The model under review builds one solid part; all positions refer to its coordinate system, in mm. A direction names the side the tool comes from. Give positions to 0.01 mm unless a question says otherwise; leave off trailing zeros. Write each loop counter-clockwise with the first axis right and the second up, starting at its lowest first coordinate (ties: lowest second). Pieces come first, ordered by that corner, then holes. Notation, with made-up numbers: (-25.75, 88) - (-18.75, 88) arc R20 ccw to (-18.75, 108) - close; hole circle Ø6 at (2.25, -25.75). An arc over 180 degrees is marked (long way). Write item = value, one per line.
```python
from build123d import *

# Parameters (mm, degrees)
F0_R     = 50.8
F0_R_2   = 47.752
F1_DEPTH = 34.036
F3_R     = 2.778125
F4_DEPTH = 12.7
F6_COUNT = 3
F6_ANGLE = 240


with BuildPart() as f1:
    # F0 (on Right) → F1 (new body, symmetric)
    with BuildSketch(Plane.YZ):
        Circle(F0_R)
        Circle(F0_R_2, mode=Mode.SUBTRACT)
    extrude(amount=F1_DEPTH, both=True)


with BuildPart() as f4:
    # F3 (on offset) → F4 (new body, symmetric)
    with BuildSketch(Plane.XY.offset(50.8)):
        with Locations((-28.575, 0)):
            Circle(F3_R)
        with Locations((28.575, 0)):
            Circle(F3_R)
    extrude(amount=F4_DEPTH, both=True)


with BuildPart() as f6_1:
    # F6: instance of F4
    add(f4.part.rotate(Axis((2.265271, 0, 0), (1, 0, 0)), 1 * F6_ANGLE / (F6_COUNT - 1)))


with BuildPart() as f6_2:
    # F6: instance of F4
    add(f4.part.rotate(Axis((2.265271, 0, 0), (1, 0, 0)), 2 * F6_ANGLE / (F6_COUNT - 1)))


with BuildPart() as f1_1:
    add(f1.part)

    # F7: cut F4, F6_2, F6_1
    add(f4.part, mode=Mode.SUBTRACT)
    add(f6_2.part, mode=Mode.SUBTRACT)
    add(f6_1.part, mode=Mode.SUBTRACT)


solid = f1_1.part
```
1. For line 1 (X direction, y = 0, z = 48.7); line 2 (Z direction, x = -12.5, y = 0); line 3 (Z direction, x = 17, y = -1.5), list the stretches that pass through material, from the lowest coordinate up. Write a range as from..to.
Findings below:
line_1 = -34.04..-31.35, -25.8..25.8, 31.35..34.04
line_2 = -50.8..-47.75, 47.75..50.8
line_3 = -50.78..-47.73, 47.73..50.78
2. Insertion check: P1, Ø1.5, axis at x = -13, y = 17.5, coming from the -Z side; P2, Ø5, axis at x = -10.5, y = -4, coming from the +Z side; P3, Ø10, axis at x = -2.5, z = -16, coming from the +Y side. Each pin has a flat end and moves straight along its axis. Give the tip position at first contact, or say it passes through.
Findings below:
P1 = -47.96
P2 = 50.78
P3 = 49.59
3. Take a section at B-B on y = 0. Give the boundary of the cut face in (x, z).
Findings below:
outline = (-34.04, -50.8) - (34.04, -50.8) - (34.04, -47.75) - (-34.04, -47.75) - close; (-34.04, 47.75) - (-31.35, 47.75) - (-31.35, 50.8) - (-34.04, 50.8) - close; (-25.8, 47.75) - (25.8, 47.75) - (25.8, 50.8) - (-25.8, 50.8) - close; (31.35, 47.75) - (34.04, 47.75) - (34.04, 50.8) - (31.35, 50.8) - close
4. Take a section at C-C on y = -35. Give the boundary of the cut face in (x, z).
Findings below:
outline = (-34.04, -36.82) - (34.04, -36.82) - (34.04, -32.48) - (-34.04, -32.48) - close; (-34.04, 32.48) - (34.04, 32.48) - (34.04, 36.82) - (-34.04, 36.82) - close
5. Draft analysis for pull direction Z (two halves, no side actions). For faces 3 (the cylindrical face through (0.477, -11.012, -49.592)), 4 (the cylindrical face through (31.225, 42.24, -25.351)), 5 (the cylindrical face through (31.225, 0.834, 49.257)), state which applies: +Z half, -Z half, draft (parallel to the pull), parting line (faces both ways), or undercut.
Findings below:
face_3 = parting line
face_4 = undercut
face_5 = draft
6. Machinability: for faces 1 (the cylindrical face through (29.857, -41.425, -26.763)), 2 (the cylindrical face through (-26.009, -1.064, 49.256)), which of the approach directions +Z, -Z, +X, -X, +Y, -Y give a long, thin tool a straight path to every point of the face, cutting with its end or side? Answer none if there is none.
Findings below:
face_1 = none
face_2 = +Z
7. Take a section at A-A on z = 0. Give the boundary of the cut face in (x, y), and give its area (3 significant figures).
Findings below:
outline = (-34.04, -50.8) - (34.04, -50.8) - (34.04, -47.75) - (-34.04, -47.75) - close; (-34.04, 47.75) - (34.04, 47.75) - (34.04, 50.8) - (-34.04, 50.8) - close
area = 415 mm²
8. Take a section at D-D on x = -20. Give the boundary of the cut face in (y, z), and give its area (3 significant figures).
Findings below:
outline = circle Ø101.6 at (0, 0); hole circle Ø95.5 at (0, 0)
area = 944 mm²
